Design review of the part built by this model. Coordinates are the model's own, in mm. Face numbers are marked on the shaded views. A direction names the side the tool comes from. Round coordinates to 2 decimals unless told otherwise and drop trailing zeros. Loops run counter-clockwise (first coordinate to the right, second up) from the corner with the lowest first, then second, coordinate; pieces in that order, holes last. Notation, with made-up numbers: (11.25, 27.25) - (29.25, 27.25) arc R34 ccw to (29.25, 60.25) - close; hole circle Ø7 at (-12.75, 44). An arc over 180 degrees is marked (long way). Return JSON: item names as keys, results as strings. Group by question number.
(1) We need section D-D, the plane y = 24. Write out the cut boundary in (x, z).
(2) We need section A-A, the plane z = 7.25. Write out the cut boundary in (x, y).
(3) We need section B-B, the plane x = -22.25. Write out the cut boundary in (y, z).
(4) Wall thickness on L1, parallel to Y at x = 22.25, z = 2.3; L2, parallel to X at y = -0.5, z = 19.25; L3, parallel to Y at x = 21, z = 2.25: over which ranges is each line inside the solid? List them lowest first. Write a range as [from, to].
(5) The part is to be moulded in two halves that separate along X. For the marked faces 1, 2 and 3, say which applies: pulls with the +X half, pulls with the -X half, needs draft (parallel to the pull), parting line crosses it, or undercut.
(6) Clearance check with flat-ended pins moving along their axes: pin 1 (1 mm diameter, centred on x = 27.5, y = -22.5, fed in from -Z); pin 2 (4 mm diameter, centred on x = 22.25, y = 27.813, fed in from +Z); pin 3 (5 mm diameter, centred on x = 4.5, z = 11, fed in from +Y); pin 4 (9.5 mm diameter, centred on x = 7, y = 27, fed in from +Z). State where each tip first meets the part, or that it passes through.
(7) We need section C-C, the plane z = 18. Write out the cut boundary in (x, y).
(8) For the marked faces 4, 5, 6 and 7, list the 3-axis set-ups (+Z, -Z, +X, -X, +Y, -Y) from which the entire face can be reached by the end or side of a thin tool; tool diameter is ignored.
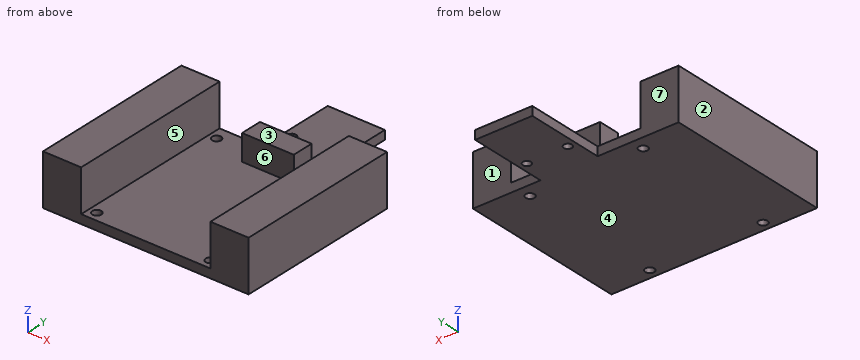
from build123d import *

# Parameters (mm, degrees)
F0_W      = 50.8
F0_H      = 66.04
F1_DEPTH  = 3.5
F2_R      = 1.75
F3_DEPTH  = 25
F4_W      = 20.32
F4_H      = 8.509
F5_DEPTH  = 10.16
F6_W      = 14.986
F6_H      = 66.04
F7_DEPTH  = 20
F9_DEPTH  = 3.5
F10_R     = 1.6
F11_DEPTH = 3.5


with BuildPart() as f1:
    # F0 (on Top) → F1 (new body)
    with BuildSketch(Plane.XY):
        Rectangle(F0_W, F0_H)
    extrude(amount=F1_DEPTH)

    # F2 (on face) → F3 (cut)
    with BuildSketch(Plane.XY.offset(3.5)):
        with Locations((-22.25, 27.813)):
            Circle(F2_R)
        with Locations((-22.25, -29.337)):
            Circle(F2_R)
        with Locations((22.25, 27.813)):
            Circle(F2_R)
        with Locations((22.25, -29.337)):
            Circle(F2_R)
    extrude(amount=-F3_DEPTH, mode=Mode.SUBTRACT)

    # F4 (on face) → F5 (join)
    with BuildSketch(Plane.XY.offset(3.5)):
        with Locations((2.66, 26.2655)):
            Rectangle(F4_W, F4_H)
    extrude(amount=F5_DEPTH)

    # F6 (on face) → F7 (join)
    with BuildSketch(Plane(origin=(0, 0, 0), x_dir=(1, 0, 0), z_dir=(0, 0, -1))):
        with Locations((32.893, 0)):
            Rectangle(F6_W, F6_H)
        with Locations((-32.893, 0)):
            Rectangle(F6_W, F6_H)
    extrude(amount=-F7_DEPTH)

    # F8 (on face) → F9 (join, through all)
    with BuildSketch(Plane.XY.offset(3.5)):
        Polygon((13.884, 64.174), (2.66, 64.174), (-8.564, 64.174), (-8.564, 33.02), (13.884, 33.02), align=None)
    extrude(amount=-F9_DEPTH)

    # F10 (on face) → F11 (cut, through all)
    with BuildSketch(Plane.XY.offset(3.5)):
        with Locations((-5.389, 43.312)):
            Circle(F10_R)
        with Locations((10.709, 43.312)):
            Circle(F10_R)
    extrude(amount=-F11_DEPTH, mode=Mode.SUBTRACT)


solid = f1.part
Solutions:
{
 "1": {"outline": "(-40.39, 0) - (40.39, 0) - (40.39, 20) - (25.4, 20) - (25.4, 3.5) - (12.82, 3.5) - (12.82, 13.66) - (-7.5, 13.66) - (-7.5, 3.5) - (-25.4, 3.5) - (-25.4, 20) - (-40.39, 20) - close"},
 "2": {"outline": "(-40.39, -33.02) - (-25.4, -33.02) - (-25.4, 33.02) - (-40.39, 33.02) - close; (-7.5, 22.01) - (12.82, 22.01) - (12.82, 30.52) - (-7.5, 30.52) - close; (25.4, -33.02) - (40.39, -33.02) - (40.39, 33.02) - (25.4, 33.02) - close"},
 "3": {"outline": "(-33.02, 0) - (-31.09, 0) - (-31.09, 3.5) - (-33.02, 3.5) - close; (-27.59, 0) - (26.06, 0) - (26.06, 3.5) - (-27.59, 3.5) - close; (29.56, 0) - (33.02, 0) - (33.02, 3.5) - (29.56, 3.5) - close"},
 "4": {"L1": "[-33.02, -31.09], [-27.59, 26.06], [29.56, 33.02]", "L2": "[-40.39, -25.4], [25.4, 40.39]", "L3": "[-33.02, -30.56], [-28.11, 26.59], [29.04, 33.02]"},
 "5": {"face 1": "needs draft", "face 2": "pulls with the -X half", "face 3": "undercut"},
 "6": {"pin 1": "z = 0", "pin 2": "z = 3.5", "pin 3": "y = 30.52", "pin 4": "z = 13.66"},
 "7": {"outline": "(-40.39, -33.02) - (-25.4, -33.02) - (-25.4, 33.02) - (-40.39, 33.02) - close; (25.4, -33.02) - (40.39, -33.02) - (40.39, 33.02) - (25.4, 33.02) - close"},
 "8": {"face 4": "-Z, +X, -X, +Y, -Y", "face 5": "+Z, +Y, -Y", "face 6": "+Z, -Y", "face 7": "+Z, -Z, -X, +Y"}
}
